```python
from build123d import *

# Parameters (mm, degrees)
SKETCH1_R               = 4.6
SKETCH1_R_2             = 2.9
BOSS_EXTRUDE1_DEPTH     = 12
CUT_EXTRUDE1_DEPTH      = 6
SKETCH3_R               = 8
BOSS_EXTRUDE2_DEPTH     = 9.45
CUT_EXTRUDE2_DEPTH      = 3.3
SKETCH5_R               = 8
BOSS_EXTRUDE3_DEPTH     = 9.45
CUT_EXTRUDE3_DEPTH      = 3.3
CUT_EXTRUDE4_DEPTH      = 3.3
CUT_EXTRUDE4_DEPTH_BACK = 3.3
CUT_EXTRUDE5_DEPTH      = 3.3
CUT_EXTRUDE5_DEPTH_BACK = 3.3


with BuildPart() as part:
    # Sketch1 → Boss-Extrude1 (new body)
    with BuildSketch(Plane(origin=(0, 0, 0), x_dir=(1, 0, 0), z_dir=(0, 1, 0))):
        with BuildLine():
            Line((-16.5, -35), (16.5, -35))
            ThreePointArc((16.5, -35), (21.449747468, -32.949747468), (23.5, -28))
            Line((23.5, -28), (23.5, 28))
            ThreePointArc((23.5, 28), (21.449747468, 32.949747468), (16.5, 35))
            Line((16.5, 35), (-16.5, 35))
            ThreePointArc((-16.5, 35), (-21.449747468, 32.949747468), (-23.5, 28))
            Line((-23.5, 28), (-23.5, -28))
            ThreePointArc((-23.5, -28), (-21.449747468, -32.949747468), (-16.5, -35))
        make_face()
        with Locations((15.5, 28)):
            Circle(SKETCH1_R, mode=Mode.SUBTRACT)
        with Locations((15.5, -28)):
            Circle(SKETCH1_R, mode=Mode.SUBTRACT)
        with Locations((0, 28)):
            Circle(SKETCH1_R_2, mode=Mode.SUBTRACT)
        with Locations((0, -28)):
            Circle(SKETCH1_R_2, mode=Mode.SUBTRACT)
        with Locations((-15.5, 28)):
            Circle(SKETCH1_R, mode=Mode.SUBTRACT)
        with Locations((-15.5, -28)):
            Circle(SKETCH1_R, mode=Mode.SUBTRACT)
    extrude(amount=BOSS_EXTRUDE1_DEPTH)

    # Sketch2 → Cut-Extrude1 (cut)
    with BuildSketch(Plane(origin=(0, 0, 0), x_dir=(1, 0, 0), z_dir=(0, 1, 0))):
        with BuildLine():
            Line((-8.006002402, -23), (8.006002402, -23))
            ThreePointArc((8.006002402, -23), (8.439015104, -22.901387819), (8.786627152, -22.625))
            ThreePointArc((8.786627152, -22.625), (12.608534281, -19.900652743), (17.291666667, -19.588702207))
            ThreePointArc((17.291666667, -19.588702207), (18.12915287, -19.387925912), (18.5, -18.610644325))
            Line((18.5, -18.610644325), (18.5, 18.610644325))
            ThreePointArc((18.5, 18.610644325), (18.129152893, 19.387925893), (17.291666727, 19.58870222))
            ThreePointArc((17.291666727, 19.58870222), (12.60853431, 19.900652732), (8.786627152, 22.625))
            ThreePointArc((8.786627152, 22.625), (8.439015104, 22.901387819), (8.006002402, 23))
            Line((8.006002402, 23), (-8.006002402, 23))
            ThreePointArc((-8.006002402, 23), (-8.439015104, 22.901387819), (-8.786627152, 22.625))
            ThreePointArc((-8.786627152, 22.625), (-12.608534281, 19.900652743), (-17.291666667, 19.588702207))
            ThreePointArc((-17.291666667, 19.588702207), (-18.12915287, 19.387925912), (-18.5, 18.610644325))
            Line((-18.5, 18.610644325), (-18.5, -18.610644325))
            ThreePointArc((-18.5, -18.610644325), (-18.129152893, -19.387925893), (-17.291666727, -19.58870222))
            ThreePointArc((-17.291666727, -19.58870222), (-12.60853431, -19.900652732), (-8.786627152, -22.625))
            ThreePointArc((-8.786627152, -22.625), (-8.439015104, -22.901387819), (-8.006002402, -23))
        make_face()
    extrude(amount=CUT_EXTRUDE1_DEPTH, mode=Mode.SUBTRACT)

    # Sketch3 → Boss-Extrude2 (add)
    with BuildSketch(Plane.XY.offset(20)):
        with BuildLine():
            Line((-24.493021315, 44.542493891), (-23.5, 12))
            Line((-23.5, 12), (23.5, 12))
            Line((23.5, 12), (3.952899906, 51.634718088))
            ThreePointArc((3.952899906, 51.634718088), (-13.128760739, 59.554452772), (-24.493021315, 44.542493891))
        make_face()
        with Locations((-9.5, 45)):
            Circle(SKETCH3_R, mode=Mode.SUBTRACT)
    extrude(amount=-BOSS_EXTRUDE2_DEPTH)

    # Sketch4 → Cut-Extrude2 (cut)
    with BuildSketch(Plane.XY.offset(20)):
        with BuildLine():
            Line((-19.168267115, 33.976179837), (-18.527256585, 12.969499593))
            ThreePointArc((-18.527256585, 12.969499593), (-18.223961586, 12.282190691), (-17.527721831, 12))
            Line((-17.527721831, 12), (16.316811337, 12))
            ThreePointArc((16.316811337, 12), (17.166021129, 12.471944387), (17.213671331, 13.442314539))
            Line((17.213671331, 13.442314539), (4.211894935, 39.805393442))
            ThreePointArc((4.211894935, 39.805393442), (3.293145866, 40.362839309), (2.399675303, 39.765716124))
            ThreePointArc((2.399675303, 39.765716124), (-6.355074026, 32.386140931), (-17.549537192, 34.791917369))
            ThreePointArc((-17.549537192, 34.791917369), (-18.618756227, 34.899696772), (-19.168267115, 33.976179837))
        make_face()
    extrude(amount=-CUT_EXTRUDE2_DEPTH, mode=Mode.SUBTRACT)

    # Sketch5 → Boss-Extrude3 (add)
    with BuildSketch(Plane.XY.offset(-20)):
        with BuildLine():
            Line((-24.493021315, 44.542493891), (-23.5, 12))
            Line((-23.5, 12), (23.5, 12))
            Line((23.5, 12), (3.952899906, 51.634718088))
            ThreePointArc((3.952899906, 51.634718088), (-13.128760739, 59.554452772), (-24.493021315, 44.542493891))
        make_face()
        with Locations((-9.5, 45)):
            Circle(SKETCH5_R, mode=Mode.SUBTRACT)
    extrude(amount=BOSS_EXTRUDE3_DEPTH)

    # Sketch6 → Cut-Extrude3 (cut)
    with BuildSketch(Plane.XY.offset(-20)):
        with BuildLine():
            Line((-19.168267115, 33.976179837), (-18.527256585, 12.969499593))
            ThreePointArc((-18.527256585, 12.969499593), (-18.223961586, 12.282190691), (-17.527721831, 12))
            Line((-17.527721831, 12), (16.316811337, 12))
            ThreePointArc((16.316811337, 12), (17.166021129, 12.471944387), (17.213671331, 13.442314539))
            Line((17.213671331, 13.442314539), (4.211894935, 39.805393442))
            ThreePointArc((4.211894935, 39.805393442), (3.293145866, 40.362839309), (2.399675303, 39.765716124))
            ThreePointArc((2.399675303, 39.765716124), (-6.355074026, 32.386140931), (-17.549537192, 34.791917369))
            ThreePointArc((-17.549537192, 34.791917369), (-18.618756227, 34.899696772), (-19.168267115, 33.976179837))
        make_face()
    extrude(amount=CUT_EXTRUDE3_DEPTH, mode=Mode.SUBTRACT)

    # Sketch7 → Cut-Extrude4 (cut, two sides)
    with BuildSketch(Plane.XY.offset(20)) as cut_extrude4_sk:
        with BuildLine():
            Line((-7.35, 30.15), (-7.35, 45))
            Line((-7.35, 45), (-11.65, 45))
            Line((-11.65, 45), (-11.65, 30.15))
            ThreePointArc((-11.65, 30.15), (-9.5, 28), (-7.35, 30.15))
        make_face()
    extrude(amount=CUT_EXTRUDE4_DEPTH, mode=Mode.SUBTRACT)
    extrude(cut_extrude4_sk.sketch, amount=-CUT_EXTRUDE4_DEPTH_BACK, mode=Mode.SUBTRACT)

    # Sketch8 → Cut-Extrude5 (cut, two sides)
    with BuildSketch(Plane.XY.offset(-20)) as cut_extrude5_sk:
        with BuildLine():
            Line((-7.35, 30.15), (-7.35, 45))
            Line((-7.35, 45), (-11.65, 45))
            Line((-11.65, 45), (-11.65, 30.15))
            ThreePointArc((-11.65, 30.15), (-9.5, 28), (-7.35, 30.15))
        make_face()
    extrude(amount=CUT_EXTRUDE5_DEPTH, mode=Mode.SUBTRACT)
    extrude(cut_extrude5_sk.sketch, amount=-CUT_EXTRUDE5_DEPTH_BACK, mode=Mode.SUBTRACT)


solid = part.part
```
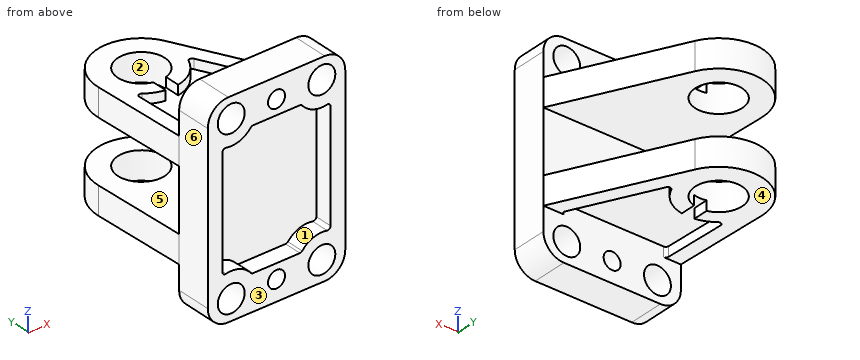
For this review, take the finished solid that the model builds, in its own axes (mm). Face numbers are marked on the shaded views. A direction names the side the tool comes from. Give positions to 0.01 mm unless a question says otherwise; leave off trailing zeros. Write each loop counter-clockwise with the first axis right and the second up, starting at its lowest first coordinate (ties: lowest second). Pieces come first, ordered by that corner, then holes. Notation, with made-up numbers: M 51,18 L 60,18 A20 cw 60,35 Z; hole C 78.5,22.5 d7. An arc over 180 degrees is marked long. Answer as a JSON object with one key per item and string values. Group by question number.
Item 1: For pin 1 Ø6 at (y, z) = (3.5, -6.5) entering from -X; pin 2 Ø14.5 at (x, y) = (4, 27.5) entering from -Z; pin 3 Ø2.5 at (y, z) = (35, -17.5) entering from +X; pin 4 Ø9.5 at (x, y) = (-9.5, 45) entering from +Z, all flat-tipped, find the tip position at first contact; note any pin that passes through.
Item 2: Tool access review of the marked faces 4, 5 and 6: name each direction out of +Z, -Z, +X, -X, +Y, -Y from which nothing blocks a thin tool from reaching the whole face with its end or side.
Item 3: For probe 1 along X at (y, z) = (9, -28); probe 2 along Y at (x, z) = (-9, -17.5); probe 3 along Z at (x, y) = (-7, 12.5), list the stretches that pass through material, from the lowest coordinate up. Write a range as [from, to].
Item 4: Draft analysis for pull direction Y (two halves, no side actions). For the marked faces 1, 2 and 3, state which applies: +Y half, -Y half, draft (parallel to the pull), parting line (faces both ways), or undercut.
Item 5: Consider section A-A on z = 13.5. Write out the cut boundary in (x, y), plus the area to 3 significant figures.
Item 6: Consider section D-D on y = 16. Write out the cut boundary in (x, z), plus the area to 3 significant figures.
Item 7: Consider section C-C on x = 0. Write out the cut boundary in (y, z), plus the area to 3 significant figures.
Item 8: Consider section B-B on y = 46.5. Write out the cut boundary in (x, z), plus the area to 3 significant figures.
Check result:
{
 "1": {"pin 1": "stops at x = -23.5", "pin 2": "stops at z = -20", "pin 3": "stops at x = 12.77", "pin 4": "passes through"},
 "2": {"face 4": "-Z, +X, -X, +Y", "face 5": "+X, -X, +Y", "face 6": "+Z, -Z, -X, -Y"},
 "3": {"probe 1": "x = [-23.5, -20.1], [-10.9, -2.9], [2.9, 10.9], [20.1, 23.5]", "probe 2": "y = [6, 12], [52.98, 59.99]", "probe 3": "z = [-16.7, -10.55], [10.55, 16.7]"},
 "4": {"face 1": "draft", "face 2": "undercut", "face 3": "-Y half"},
 "5": {"outline": "M -24.49,44.54 L -23.5,12 L -23.5,0 L -18.5,0 L -18.5,6 L 18.5,6 L 18.5,0 L 23.5,0 L 23.5,12 L 3.95,51.63 A15 ccw Z; hole C -9.5,45 d16", "area": "1,800 mm^2"},
 "6": {"outline": "M -23.62,-20 L -18.62,-20 L -18.62,-16.7 L 15.95,-16.7 L 15.95,-20 L 21.53,-20 L 21.53,-10.55 L -23.62,-10.55 Z; M -23.62,10.55 L 21.53,10.55 L 21.53,20 L 15.95,20 L 15.95,16.7 L -18.62,16.7 L -18.62,20 L -23.62,20 Z", "area": "625 mm^2"},
 "7": {"outline": "M 0,-35 L 12,-35 L 12,-30.9 L 0,-30.9 Z; M 0,-25.1 L 12,-25.1 L 12,-16.7 L 36.13,-16.7 L 36.13,-20 L 56.61,-20 L 56.61,-10.55 L 12,-10.55 L 12,10.55 L 56.61,10.55 L 56.61,20 L 36.13,20 L 36.13,16.7 L 12,16.7 L 12,25.1 L 0,25.1 L 0,23 L 6,23 L 6,-23 L 0,-23 Z; M 0,30.9 L 12,30.9 L 12,35 L 0,35 Z", "area": "1,110 mm^2"},
 "8": {"outline": "M -24.42,-20 L -17.36,-20 L -17.36,-10.55 L -24.42,-10.55 Z; M -24.42,10.55 L -17.36,10.55 L -17.36,20 L -24.42,20 Z; M -1.64,-20 L 6.49,-20 L 6.49,-10.55 L -1.64,-10.55 Z; M -1.64,10.55 L 6.49,10.55 L 6.49,20 L -1.64,20 Z", "area": "287 mm^2"}
}
